from build123d import *

# Parameters (mm, degrees)
SKETCH_W        = 50
SKETCH_H        = 48
PAD_DEPTH       = 11
CHAMFER_1_ANGLE = 30
CHAMFER_1_SIZE  = 9
CHAMFER_2_ANGLE = 30
CHAMFER_2_SIZE  = 9
FILLET_R        = 3
PAD001_DEPTH    = 0.5
SKETCH002_R     = 3.175
POCKET_DEPTH    = 11.501
POCKET001_DEPTH = 6


with BuildPart() as part:
    # Sketch → Pad (new body)
    with BuildSketch(Plane.XY):
        with Locations((25, 24)):
            Rectangle(SKETCH_W, SKETCH_H)
    extrude(amount=PAD_DEPTH)

    # Chamfer 1
    chamfer_1_edges = [part.edges().sort_by_distance(p)[0] for p in [
        (25, 0, 11),
    ]]
    chamfer_1_side = part.faces().sort_by_distance((25, 0, 5.5))[0]
    chamfer(chamfer_1_edges, length=CHAMFER_1_SIZE, angle=CHAMFER_1_ANGLE, reference=chamfer_1_side)

    # Chamfer 2
    chamfer_2_edges = [part.edges().sort_by_distance(p)[0] for p in [
        (25, 48, 11),
    ]]
    chamfer_2_side = part.faces().sort_by_distance((25, 48, 5.5))[0]
    chamfer(chamfer_2_edges, length=CHAMFER_2_SIZE, angle=CHAMFER_2_ANGLE, reference=chamfer_2_side)

    # Fillet
    fillet_edges = [part.edges().sort_by_distance(p)[0] for p in [
        (50, 2.598076, 6.5),
        (50, 0, 1),
        (50, 45.401924, 6.5),
        (50, 48, 1),
        (0, 45.401924, 6.5),
        (0, 48, 1),
        (0, 2.598076, 6.5),
        (0, 0, 1),
    ]]
    fillet(fillet_edges, radius=FILLET_R)

    # Sketch001 (on DatumPlane) → Pad001 (join)
    with BuildSketch(Plane.XY.offset(11)):
        with BuildLine():
            Line((7.5, 39.5), (42.5, 39.5))
            ThreePointArc((42.5, 29.5), (47.5, 34.5), (42.5, 39.5))
            Line((42.5, 29.5), (7.5, 29.5))
            ThreePointArc((7.5, 39.5), (2.5, 34.5), (7.5, 29.5))
        make_face()
        with BuildLine():
            Line((7.5, 18.5), (42.5, 18.5))
            ThreePointArc((42.5, 8.5), (47.5, 13.5), (42.5, 18.5))
            Line((42.5, 8.5), (7.5, 8.5))
            ThreePointArc((7.5, 18.5), (2.5, 13.5), (7.5, 8.5))
        make_face()
    extrude(amount=PAD001_DEPTH)

    # Sketch002 → Pocket (cut, through all)
    with BuildSketch(Plane.XY):
        with Locations((25, 24)):
            Circle(SKETCH002_R)
    extrude(amount=POCKET_DEPTH, mode=Mode.SUBTRACT)

    # Sketch003 → Pocket001 (cut)
    with BuildSketch(Plane.XY):
        with BuildLine():
            Line((6, 37.5), (44, 37.5))
            ThreePointArc((46, 35.5), (45.414214, 36.914214), (44, 37.5))
            Line((46, 35.5), (46, 12.5))
            ThreePointArc((44, 10.5), (45.414214, 11.085786), (46, 12.5))
            Line((44, 10.5), (6, 10.5))
            ThreePointArc((4, 12.5), (4.585786, 11.085786), (6, 10.5))
            Line((4, 12.5), (4, 35.5))
            ThreePointArc((6, 37.5), (4.585786, 36.914214), (4, 35.5))
        make_face()
    extrude(amount=POCKET001_DEPTH, mode=Mode.SUBTRACT)


solid = part.part
The listing builds one solid part. Answer for the finished solid, in the listing's coordinates (mm). A direction names the side the tool comes from. Round coordinates to 2 decimals unless told otherwise and drop trailing zeros. Write each loop counter-clockwise with the first axis right and the second up, starting at its lowest first coordinate (ties: lowest second). Pieces come first, ordered by that corner, then holes. Notation, with made-up numbers: (-23, 8) - (7, 8) arc R22 ccw to (7, 15) - close; hole circle Ø11 at (-2, -5). An arc over 180 degrees is marked (long way). Use one line per item in the form item = value. Start each with the question number.
Item 1: Find the intervals of material crossed by line 1 (X direction, y = 24, z = 8.25) (3 decimals); line 2 (X direction, y = 25.5, z = 5); line 3 (Y direction, x = 16.5, z = 1.5), in increasing order. Write a range as [from, to].
Item 2: Flat-ended cylindrical pins translate along their axes: pin 1 Ø8 at (x, y) = (17.5, 27) entering from -Z; pin 2 Ø5 at (x, z) = (26, 3) entering from +Y; pin 3 Ø0.6 at (x, z) = (21, 11.5) entering from -Y; pin 4 Ø0.6 at (x, z) = (26, 11.5) entering from +Y. Find the tip coordinate at first contact, or state that the pin passes through.
Item 3: A cutting plane is placed at D-D (y = 17). Write down the section's boundary in (x, z).
Item 4: A cutting plane is placed at B-B (y = 34.5). Write down the section's boundary in (x, z), plus the area to 4 significant figures.
Item 5: A tool of negligible diameter and unlimited length cuts with its end or side. For faces 4 (the cylindrical face through (47.5, 34.4, 11.2)), 5 (the cylindrical face through (2.5, 34.6, 11.2)), 6 (the cylindrical face through (45.43, 36.9, 2.96)), 7 (the flat face through (25, 14, 11.5)), from which of +Z, -Z, +X, -X, +Y, -Y can it reach the whole face along a straight path? Write none if from no direction.
Item 6: Determine the mould class of faces 1 (the flat face through (25, 37.5, 3)), 2 (the cylindrical face through (2.5, 13.6, 11.2)), 3 (the flat face through (24.692, 45.366, 6.563)) for opening direction X: +X half, -X half, draft (parallel to the pull), parting line (faces both ways), or undercut.
Item 7: A cutting plane is placed at C-C (x = 30). Write down the section's boundary in (y, z).
Item 8: A cutting plane is placed at A-A (x = 24). Write down the section's boundary in (y, z), plus the area to 3 significant figures.
The answers:
q1.line_1 = [0, 21.825], [28.175, 50]
q1.line_2 = [0, 4], [46, 50]
q1.line_3 = [0, 10.5], [37.5, 48]
q2.pin_1 = 6
q2.pin_2 = 48
q2.pin_3 = 8.5
q2.pin_4 = 39.5
q3.outline = (0, 0) - (4, 0) - (4, 6) - (46, 6) - (46, 0) - (50, 0) - (50, 11) - (46.07, 11) - (46.07, 11.5) - (3.93, 11.5) - (3.93, 11) - (0, 11) - close
q4.outline = (0, 0) - (4, 0) - (4, 6) - (46, 6) - (46, 0) - (50, 0) - (50, 11) - (47.5, 11) - (47.5, 11.5) - (2.5, 11.5) - (2.5, 11) - (0, 11) - close
q4.area = 320.5 mm^2
q5.face_4 = +Z, +X
q5.face_5 = +Z, -X
q5.face_6 = -Z
q5.face_7 = +Z, +X, -X, +Y, -Y
q6.face_1 = undercut
q6.face_2 = -X half
q6.face_3 = draft
q7.outline = (0, 0) - (10.5, 0) - (10.5, 6) - (37.5, 6) - (37.5, 0) - (48, 0) - (48, 2) - (42.8, 11) - (39.5, 11) - (39.5, 11.5) - (29.5, 11.5) - (29.5, 11) - (18.5, 11) - (18.5, 11.5) - (8.5, 11.5) - (8.5, 11) - (5.2, 11) - (0, 2) - close
q8.outline = (0, 0) - (10.5, 0) - (10.5, 6) - (20.99, 6) - (20.99, 11) - (18.5, 11) - (18.5, 11.5) - (8.5, 11.5) - (8.5, 11) - (5.2, 11) - (0, 2) - close; (27.01, 6) - (37.5, 6) - (37.5, 0) - (48, 0) - (48, 2) - (42.8, 11) - (39.5, 11) - (39.5, 11.5) - (29.5, 11.5) - (29.5, 11) - (27.01, 11) - close
q8.area = 299 mm^2
